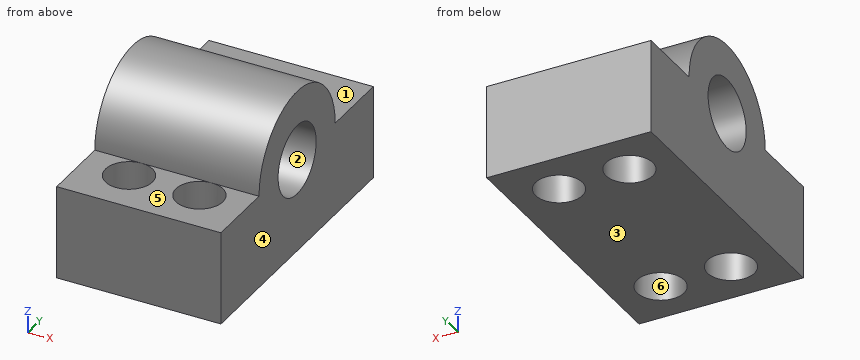
```python
from build123d import *

# Parameters (mm, degrees)
BODY_DEPTH         = 35
SKETCH2_R          = 5
FIXING_HOLES_DEPTH = 58.879184514
SKETCH3_R          = 7.5
SHAFT_HOLE_DEPTH   = 40


with BuildPart() as part:
    # Sketch1 → body (new body)
    with BuildSketch(Plane(origin=(0, 0, 0), x_dir=(0, 0, -1), z_dir=(1, 0, 0))):
        with BuildLine():
            Line((0, -30), (0, 30))
            Line((0, 30), (-20, 30))
            Line((-20, 30), (-20, 15))
            ThreePointArc((-20, 15), (-35, 0), (-20, -15))
            Line((-20, -15), (-20, -30))
            Line((-20, -30), (0, -30))
        make_face()
    extrude(amount=BODY_DEPTH)

    # Sketch2 → fixing holes (cut, through all)
    with BuildSketch(Plane.XY):
        with Locations(Location((10, 20, 0), (0, 0, 270))):
            Circle(SKETCH2_R)
        with Locations(Location((25, 20, 0), (0, 0, 270))):
            Circle(SKETCH2_R)
        with Locations(Location((10, -20, 0), (0, 0, 90))):
            Circle(SKETCH2_R)
        with Locations(Location((25, -20, 0), (0, 0, 90))):
            Circle(SKETCH2_R)
    extrude(amount=FIXING_HOLES_DEPTH, mode=Mode.SUBTRACT)

    # Sketch3 → shaft hole (cut)
    with BuildSketch(Plane(origin=(35, 0, 0), x_dir=(0, 0, -1), z_dir=(1, 0, 0))):
        with Locations((-20, 0)):
            Circle(SKETCH3_R)
    extrude(amount=-SHAFT_HOLE_DEPTH, mode=Mode.SUBTRACT)


solid = part.part
```
Geometry: final body of the model. Coordinates: model frame, mm. Face numbers are marked on the shaded views. A direction names the side the tool comes from. Give positions to 0.01 mm unless a question says otherwise; leave off trailing zeros. Order: outer loops, then holes, each group sorted by start corner. A loop starts at its lowest first (then second) coordinate and runs counter-clockwise, first axis right, second up. Notation, with made-up numbers: M -30,12 L 12,12 A21 cw 12,40 Z; hole C -9.5,-12 d4. An arc over 180 degrees is marked long. Answer as CSV lines item,"result". Start each with the question number.
1) Cut plane A-A (y = 0). Output: boundary loops of the cut face in (x, z).
2) Cut plane B-B (x = 23). Output: boundary loops of the cut face in (y, z).
3) Cut plane C-C (y = -20). Output: boundary loops of the cut face in (x, z).
4) Cut plane D-D (x = 18.5). Output: boundary loops of the cut face in (y, z), then the cut area to 3 significant figures.
5) Line query: line 1 (X direction, y = -20, z = 15.5); line 2 (Y direction, x = 25, z = 8); line 3 (Y direction, x = 25, z = 14). Output: solid intervals per line, ascending. Write a range as from..to.
6) First-contact query: P1, Ø1, axis at x = 10, y = -11, coming from the +Z side; P2, Ø13, axis at x = 10, y = -20, coming from the +Z side; P3, Ø6, axis at x = 27, z = 26, coming from the +Y side. Flat tips, straight axial feed; report the tip coordinate or a pass-through.
7) Mould query, pull axis Z, two halves, no side actions, for the marked faces 1, 2, 3 and 4. Classes: +Z half, -Z half, draft (parallel to the pull), parting line (faces both ways), or undercut.
8) Set-up query: the marked faces 5 and 6. Return all of +Z, -Z, +X, -X, +Y, -Y with unobstructed straight access to the full face (end or side cutting, diameter ignored); none if empty.
Findings below:
1,outline,"M 0,0 L 35,0 L 35,12.5 L 0,12.5 Z; M 0,27.5 L 35,27.5 L 35,35 L 0,35 Z"
2,outline,"M -30,0 L -24.58,0 L -24.58,20 L -30,20 Z; M -15.42,0 L 15.42,0 L 15.42,20 L 15,20 A15 ccw -15,20 L -15.42,20 Z; M 24.58,0 L 30,0 L 30,20 L 24.58,20 Z; hole C 0,20 d15"
3,outline,"M 0,0 L 5,0 L 5,20 L 0,20 Z; M 15,0 L 20,0 L 20,20 L 15,20 Z; M 30,0 L 35,0 L 35,20 L 30,20 Z"
4,outline,"M -30,0 L 30,0 L 30,20 L 15,20 A15 ccw -15,20 L -30,20 Z; hole C 0,20 d15"
4,area,"1,380 mm²"
5,line 1,"x = 0..5, 15..20, 30..35"
5,line 2,"y = -30..-25, -15..15, 25..30"
5,line 3,"y = -30..-25, -15..-4.5, 4.5..15, 25..30"
6,P1,"stops at z = 30.71"
6,P2,"stops at z = 26.54"
6,P3,"stops at y = 14.7"
7,face 1,"+Z half"
7,face 2,"undercut"
7,face 3,"-Z half"
7,face 4,"draft"
8,face 5,"+Z, +X, -X, -Y"
8,face 6,"+Z, -Z"
